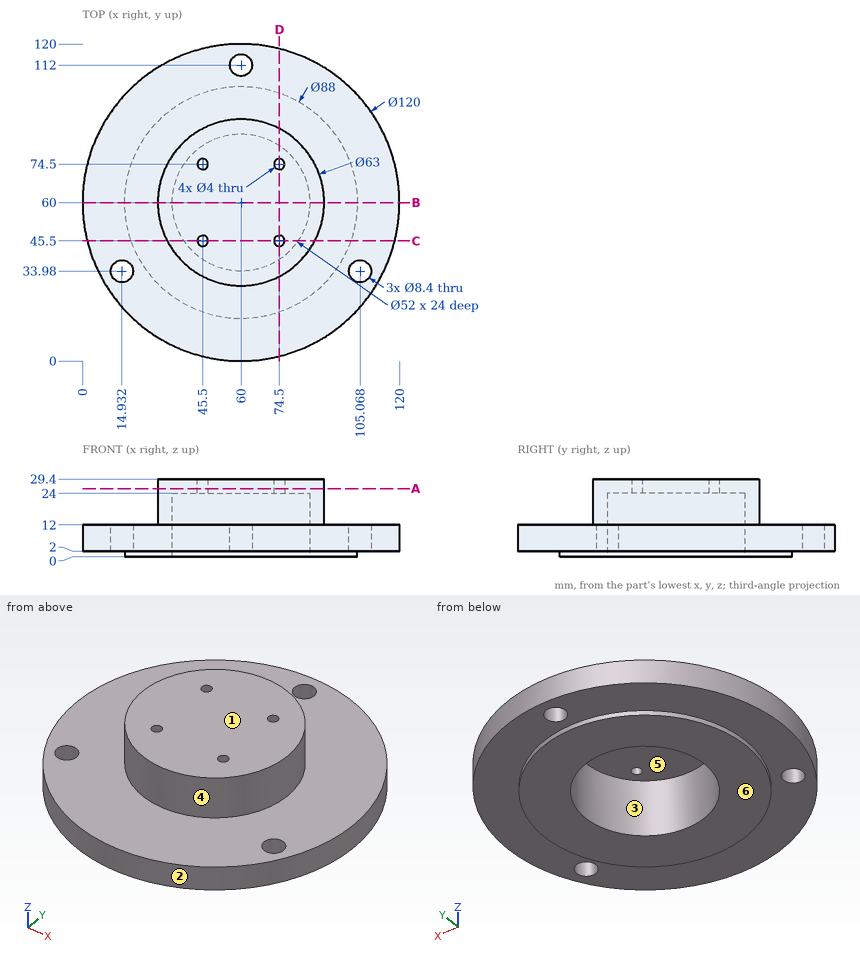
Print and shaded views of the part. All mm, measured from the part's lowest x, y and z. A direction names the side the tool comes from. Give positions to 0.01 mm unless a question says otherwise; leave off trailing zeros. Order: outer loops, then holes, each group sorted by start corner. A loop starts at its lowest first (then second) coordinate and runs counter-clockwise, first axis right, second up. Notation, with made-up numbers: (76.5, 61) - (118.5, 61) arc R25 cw to (118.5, 79) - close; hole circle Ø4 at (70.5, 18.5). An arc over 180 degrees is marked (long way). One line per item, written item: value.
Item 1: Slice it at B-B (y = 60). List the corners of the cut face in (x, z), then the cut area to 3 significant figures.
Response values:
outline: (0, 2) - (16, 2) - (16, 0) - (34, 0) - (34, 24) - (86, 24) - (86, 0) - (104, 0) - (104, 2) - (120, 2) - (120, 12) - (91.5, 12) - (91.5, 29.4) - (28.5, 29.4) - (28.5, 12) - (0, 12) - close
area: 1,220 mm2
Item 2: Slice it at C-C (y = 45.5). List the corners of the cut face in (x, z), then the cut area to 3 significant figures.
Response values:
outline: (1.78, 2) - (18.46, 2) - (18.46, 0) - (38.42, 0) - (38.42, 24) - (43.5, 24) - (43.5, 29.4) - (32.04, 29.4) - (32.04, 12) - (1.78, 12) - close; (47.5, 24) - (72.5, 24) - (72.5, 29.4) - (47.5, 29.4) - close; (76.5, 24) - (81.58, 24) - (81.58, 0) - (101.54, 0) - (101.54, 2) - (118.22, 2) - (118.22, 12) - (87.96, 12) - (87.96, 29.4) - (76.5, 29.4) - close
area: 1,220 mm2
Item 3: Slice it at A-A (z = 25.75). List the corners of the cut face in (x, y).
Response values:
outline: circle Ø63 at (60, 60); hole circle Ø4 at (45.5, 45.5); hole circle Ø4 at (45.5, 74.5); hole circle Ø4 at (74.5, 45.5); hole circle Ø4 at (74.5, 74.5)
Item 4: Wall check: line 1 (Y direction, x = 60, z = 6.25); line 2 (Y direction, x = 74.5, z = 26.4); line 3 (Z direction, x = 108, y = 75). Give the ranges that are in metal, low to high.
Response values:
line 1: 0 to 34, 86 to 107.8, 116.2 to 120
line 2: 32.04 to 43.5, 47.5 to 72.5, 76.5 to 87.96
line 3: 2 to 12
Item 5: Pin check, flat tips, straight feed: pin 1 Ø1.5 at (x, z) = (87, 9.5) entering from -Y; pin 2 Ø13.5 at (x, y) = (105.068, 33.98) entering from +Z; pin 3 Ø12 at (x, z) = (80.5, 16.5) entering from +Y. Stop position of each tip, or through.
Response values:
pin 1: y = 6.05
pin 2: z = 12
pin 3: y = 117.68
Item 6: Tool access for the marked faces 4, 5 and 6: list every direction of +Z, -Z, +X, -X, +Y, -Y with a clear straight run to the whole face (end or side of a thin tool).
Response values:
face 4: +Z
face 5: -Z
face 6: -Z, +X, -X, +Y, -Y
Item 7: Two-plate mould, pull along Y, no slides. Class the marked faces 1, 2 and 3: released by +Y, released by -Y, zero draft, split by the parting line, or undercut.
Response values:
face 1: zero draft
face 2: split by the parting line
face 3: undercut
